Can you work these out from the drawing? Everything is in mm from the part's minimum corner. Coordinates: 2 decimals unless noted, no trailing zeros. Write each loop counter-clockwise with the first axis right and the second up, starting at its lowest first coordinate (ties: lowest second). Pieces come first, ordered by that corner, then holes. Notation, with made-up numbers: M 52.5,14 L 88.5,14 A7 cw 88.5,18 Z; hole C 80,-14.5 d2. An arc over 180 degrees is marked long. Write item = value, one per line.
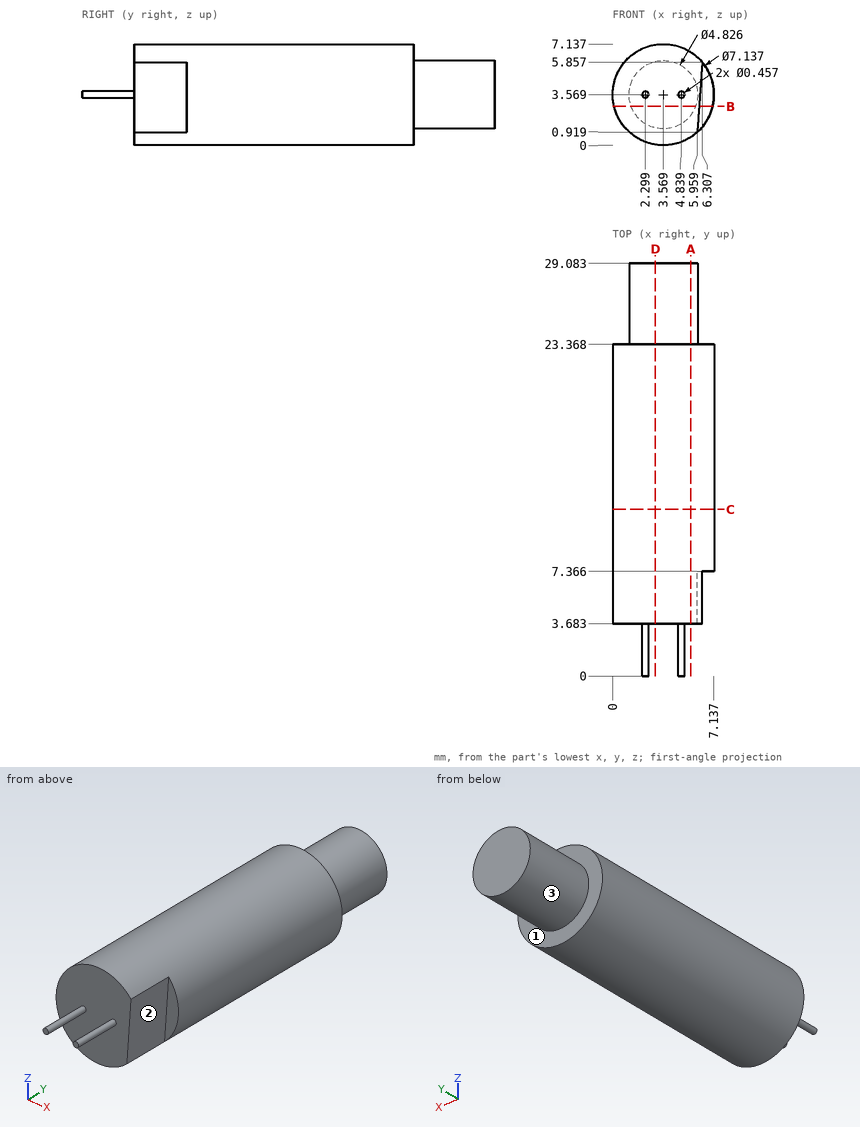
Item 1: Imagine slicing it at C-C (y = 11.75). Write out the boundary of the cut face in (x, z), and give its area (3 significant figures).
Numbers:
outline = C 3.57,3.57 d7.14
area = 40.0 mm²
Item 2: Imagine slicing it at B-B (z = 2.75). Write out the boundary of the cut face in (x, y) (1 decimal).
Numbers:
outline = M 0.1,3.7 L 6.1,3.7 L 6.1,7.4 L 7,7.4 L 7,23.4 L 5.8,23.4 L 5.8,29.1 L 1.3,29.1 L 1.3,23.4 L 0.1,23.4 Z
Item 3: If I drill on line 1 along Y through (x, z) = (6, 4.5); line 2 along Y through (x, z) = (2.5, 1.5); line 3 along Z through (x, y) = (6.5, 22.5) (1 decimal), over which ranges is the centre line in solid material (lowest first)?
Numbers:
line_1 = 3.68 to 23.37
line_2 = 3.68 to 29.08
line_3 = 1.5 to 5.6
Item 4: Imagine slicing it at D-D (x = 3). Write out the boundary of the cut face in (y, z) (1 decimal).
Numbers:
outline = M 3.7,0 L 23.4,0 L 23.4,1.2 L 29.1,1.2 L 29.1,5.9 L 23.4,5.9 L 23.4,7.1 L 3.7,7.1 Z
Item 5: I'm going to push flat-ended pins straight in: P1, Ø4, axis at x = 2.5, z = 6.5, coming from the +Y side; P2, Ø1, axis at y = 22.5, z = 6, coming from the +X side; P3, Ø0.6, axis at x = 6.5, z = 2.5, coming from the -Y side; P4, Ø2, axis at y = 5.5, z = 1.5, coming from the -X side. Where does each tip first touch, or does it pass through?
Numbers:
P1 = 29.08
P2 = 6.57
P3 = 7.37
P4 = 0.16
Item 6: Imagine slicing it at A-A (x = 5.5). Write out the boundary of the cut face in (y, z) (1 decimal).
Numbers:
outline = M 3.7,0.6 L 23.4,0.6 L 23.4,2.1 L 29.1,2.1 L 29.1,5 L 23.4,5 L 23.4,6.6 L 3.7,6.6 Z
Item 7: If we mould it in two halves opening along Z, with no side actions, what happens to the marked faces 1, 2 and 3? For each: pulls with the +Z half, pulls with the -Z half, needs draft (parallel to the pull), parting line crosses it, or undercut.
Numbers:
face_1 = needs draft
face_2 = pulls with the -Z half
face_3 = parting line crosses it
